Design review of the part shown in the three views and the two pictorial views. Dimensions are in mm from the part's minimum x, y and z. Give positions to 0.01 mm unless a question says otherwise; leave off trailing zeros. Order: outer loops, then holes, each group sorted by start corner. A loop starts at its lowest first (then second) coordinate and runs counter-clockwise, first axis right, second up.
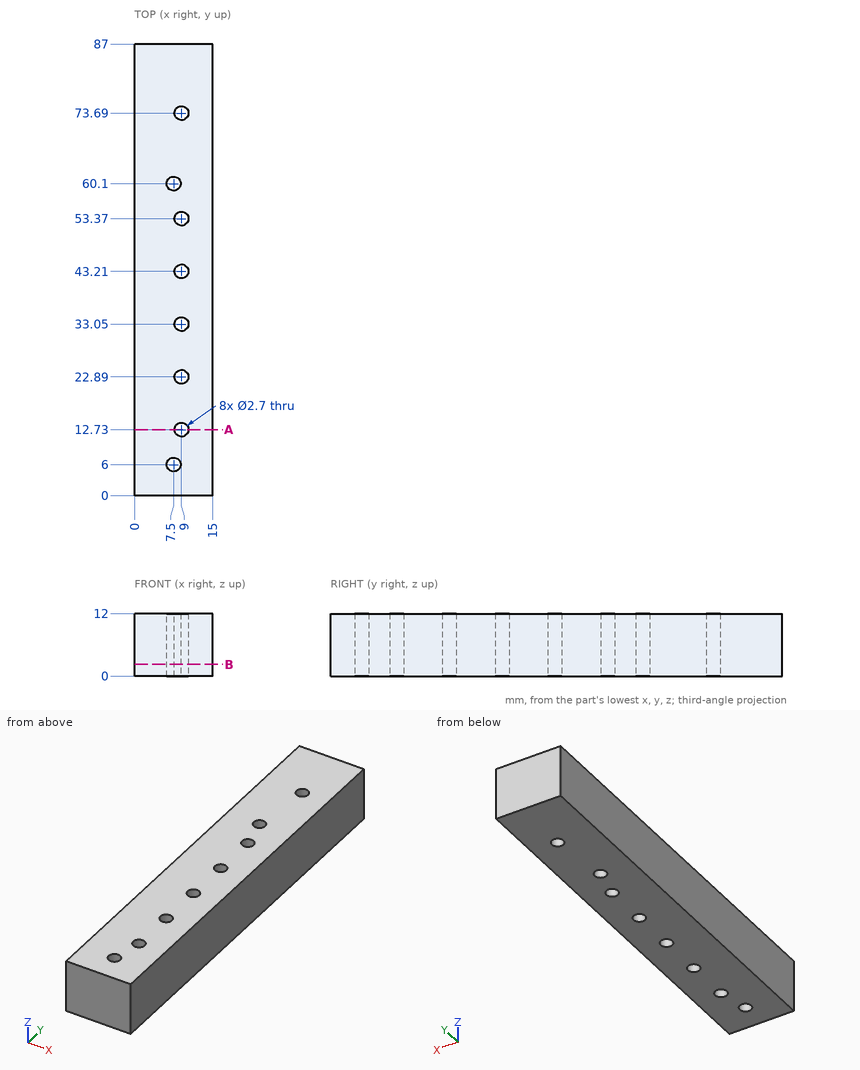
1) To check wall thickness, follow line 1 (Y direction, x = 7.5, z = 4.75); line 2 (X direction, y = 60, z = 3.75); line 3 (X direction, y = 33, z = 9). State the ranges of each line that lie inside material, in increasing order.
Answer sheet:
line 1: y = 0 to 4.65, 7.35 to 58.75, 61.45 to 87
line 2: x = 0 to 6.15, 8.85 to 15
line 3: x = 0 to 7.65, 10.35 to 15
2) Clearance check with flat-ended pins moving along their axes: pin 1 (2 mm diameter, centred on x = 7.5, y = 60.1, fed in from +Z); pin 2 (4 mm diameter, centred on x = 12.5, y = 34.5, fed in from -Z). State where each tip first meets the part, or that it passes through.
Answer sheet:
pin 1: passes through
pin 2: stops at z = 0
3) We need section A-A on y = 12.73. Give the boundary of the cut face in (x, z), then the cut area to 3 significant figures.
Answer sheet:
outline: (0, 0) - (7.65, 0) - (7.65, 12) - (0, 12) - close; (10.35, 0) - (15, 0) - (15, 12) - (10.35, 12) - close
area: 148 mm2
4) We need section B-B on z = 2.25. Count the separate pieces of the cut face and the enclosed holes in it, then the cut area to 3 significant figures.
Answer sheet:
separate pieces: 1
enclosed holes: 8
area: 1,260 mm2
